from build123d import *


with BuildPart() as part:
    # 草图1 → 旋转1 (revolve)
    with BuildSketch(Plane.XY):
        Polygon((30, 0), (-30, 0), (-30, 4), (-32, 4), (-32, 0), (-38, 0), (-38, 4), (-40, 4), (-40, 0), (-40, -2), (40, -2), (40, 0), (40, 4), (38, 4), (38, 0), (32, 0), (32, 4), (30, 4), align=None)
    revolve(axis=Axis((-40, -2, 0), (1, 0, 0)))


solid = part.part
Build history of the part. All positions in model axes, mm. A direction names the side the tool comes from. Round coordinates to 2 decimals unless told otherwise and drop trailing zeros. Write each loop counter-clockwise with the first axis right and the second up, starting at its lowest first coordinate (ties: lowest second). Pieces come first, ordered by that corner, then holes. Notation, with made-up numbers: M -26,8.5 L 8,8.5 A17 ccw 8,32.5 Z; hole C 18.5,10.5 d10. An arc over 180 degrees is marked long. Answer as a JSON object with one key per item and string values. Group by question number.
(1) Cut at C-C (y = -2). Give the cut face in (x, z), and give its area (3 significant figures).
(2) Cut at A-A (y = -7). Give the cut face in (x, z), and give its area (3 significant figures).
(3) Cut at D-D (z = -3). Give the cut face in (x, y).
(4) Cut at B-B (z = 0). Give the cut face in (x, y), and give its area (3 significant figures).
(5) Drill centre lines: L1, parallel to X at y = -4.25, z = -4.25; L2, parallel to Z at x = -22, y = -2.25; L3, parallel to Z at x = -19, y = -0.5. Where is each one in solid material? Low to high.
(6) Which spindle directions (+Z, -Z, +X, -X, +Y, -Y) get a long thin tool onto all of the face, cutting with end or side? Do faces 5 (the cylindrical face through (-39.014, 3.723, 1.802)), 6 (the flat face through (30, 1, 0)). Say none if no direction does.
(7) Mould opens along X. For faces 1 (the cylindrical face through (38.986, 3.723, 1.802)), 2 (the flat face through (-38, -5, 0)), 3 (the flat face through (40, -2, 0)), 4 (the flat face through (-40, -2, 0)) say: pulls with the +X half, pulls with the -X half, needs draft (parallel to the pull), parting line crosses it, or undercut.
Responses:
{
 "1": {"outline": "M -40,-6 L -38,-6 L -38,-2 L -32,-2 L -32,-6 L -30,-6 L -30,-2 L 30,-2 L 30,-6 L 32,-6 L 32,-2 L 38,-2 L 38,-6 L 40,-6 L 40,6 L 38,6 L 38,2 L 32,2 L 32,6 L 30,6 L 30,2 L -30,2 L -30,6 L -32,6 L -32,2 L -38,2 L -38,6 L -40,6 Z", "area": "384 mm2"},
 "2": {"outline": "M -40,-3.32 L -38,-3.32 L -38,3.32 L -40,3.32 Z; M -32,-3.32 L -30,-3.32 L -30,3.32 L -32,3.32 Z; M 30,-3.32 L 32,-3.32 L 32,3.32 L 30,3.32 Z; M 38,-3.32 L 40,-3.32 L 40,3.32 L 38,3.32 Z", "area": "53.1 mm2"},
 "3": {"outline": "M -40,-7.2 L -38,-7.2 L -38,3.2 L -40,3.2 Z; M -32,-7.2 L -30,-7.2 L -30,3.2 L -32,3.2 Z; M 30,-7.2 L 32,-7.2 L 32,3.2 L 30,3.2 Z; M 38,-7.2 L 40,-7.2 L 40,3.2 L 38,3.2 Z"},
 "4": {"outline": "M -40,-8 L -38,-8 L -38,-4 L -32,-4 L -32,-8 L -30,-8 L -30,-4 L 30,-4 L 30,-8 L 32,-8 L 32,-4 L 38,-4 L 38,-8 L 40,-8 L 40,4 L 38,4 L 38,0 L 32,0 L 32,4 L 30,4 L 30,0 L -30,0 L -30,4 L -32,4 L -32,0 L -38,0 L -38,4 L -40,4 Z", "area": "384 mm2"},
 "5": {"L1": "x = -40 to -38, -32 to -30, 30 to 32, 38 to 40", "L2": "z = -1.98 to 1.98", "L3": "z = -1.32 to 1.32"},
 "6": {"face 5": "+X, -X", "face 6": "none"},
 "7": {"face 1": "needs draft", "face 2": "undercut", "face 3": "pulls with the +X half", "face 4": "pulls with the -X half"}
}
